Geometry: final body of the model. Coordinates: model frame, mm. A direction names the side the tool comes from. Coordinates: 2 decimals unless noted, no trailing zeros. Loops run counter-clockwise (first coordinate to the right, second up) from the corner with the lowest first, then second, coordinate; pieces in that order, holes last. Notation, with made-up numbers: (-40, 6) - (1, 6) arc R17 ccw to (1, 19) - close; hole circle Ø4 at (-10, -24). An arc over 180 degrees is marked (long way). Put each result on its own line as item: value. Start each with the question number.
1) Reachability of faces 4 (the flat face through (10, 3, 7)), 5 (the flat face through (20.5, 0, 8)), 6 (the flat face through (10, -3, 7)) from +Z, -Z, +X, -X, +Y, -Y: full face, straight path, thin tool, end or side. Return the list, or none.
2) Section B-B on x = 10. Output: boundary loops of the cut face in (y, z), and give its area (3 significant figures).
3) Section C-C on y = 0. Output: boundary loops of the cut face in (x, z), and give its area (3 significant figures).
4) Section A-A on z = 15. Output: boundary loops of the cut face in (x, y), and give its area (3 significant figures).
5) Section D-D on z = 9.5. Output: boundary loops of the cut face in (x, y), and give its area (3 significant figures).
6) Draft query along X for faces 1 (the cylindrical face through (13.502, -9.715, 0.301)), 2 (the cylindrical face through (28.58, 0.78, 2.54)), 3 (the flat face through (31.5, 0, 2)). Return one class per face: +X half, -X half, draft (parallel to the pull), parting line (faces both ways), or undercut.
7) Material intervals for line 1 along Y through (x, z) = (10, 3.5); line 2 along Z through (x, y) = (-2.95, 0); line 3 along X through (y, z) = (2, 12.25), sorted ascending. Write a range as from..to.
8) Contact query for flat-ended pins moving along their axis: pin 1 Ø4 at (y, z) = (2.5, 18.5) entering from +X; pin 2 Ø5 at (x, y) = (6, 0.5) entering from +Z; pin 3 Ø8 at (x, z) = (15, 11.5) entering from -Y; pin 4 Ø4 at (x, y) = (10, 0) entering from -Z. Output: stop coordinate, or through.
```python
from build123d import *

# Parameters (mm, degrees)
F0_W      = 31.5
F0_H      = 20
F1_DEPTH  = 5
F2_W      = 31.5
F2_H      = 6
F3_DEPTH  = 5
F4_R      = 2.5
F5_DEPTH  = 25
F6_W      = 11.2
F6_H      = 6
F7_DEPTH  = 5
F8_R      = 2.6
F9_DEPTH  = 5
F10_R     = 2.6
F11_DEPTH = 4
F12_R     = 1


# Not quite as in the source:
# - a fillet or chamfer that OpenCascade refuses, or shapes differently, is made with other operations: its cross-section is extruded or revolved along the edge and cut away or added
# - a feature names something its author has since deleted; it is built from what else it names


with BuildPart() as f1:
    # F0 (on Top) → F1 (new body)
    with BuildSketch(Plane.XY):
        with Locations((15.75, 0)):
            Rectangle(F0_W, F0_H)
    extrude(amount=F1_DEPTH)

    # F2 (on face) → F3 (join)
    with BuildSketch(Plane.XY.offset(5)):
        with Locations((15.75, 0)):
            Rectangle(F2_W, F2_H)
    extrude(amount=F3_DEPTH)

    # F4 (on face) → F5 (cut)
    with BuildSketch(Plane.XY.offset(10)):
        with Locations((10, 0)):
            Circle(F4_R)
    extrude(amount=-F5_DEPTH, mode=Mode.SUBTRACT)

    # F6 (on face) → F7 (cut, through all)
    with BuildSketch(Plane.XY.offset(10)):
        with Locations((26.1, 0)):
            Rectangle(F6_W, F6_H)
    extrude(amount=-F7_DEPTH, mode=Mode.SUBTRACT)

    # F8 (on face) → F9 (cut, through all)
    with BuildSketch(Plane.XY.offset(5)):
        with Locations((26.1, 0)):
            Circle(F8_R)
    extrude(amount=-F9_DEPTH, mode=Mode.SUBTRACT)

    # F10 (on face) → F11 (join)
    with BuildSketch(Plane(origin=(0, 0, 0), x_dir=(0, -1, 0), z_dir=(-1, 0, 0))):
        Polygon((-10, 25), (-10, 5), (-3, 5), (-3, 10), (3, 10), (3, 5), (10, 5), (10, 25), align=None)
        with Locations((0, 15)):
            Circle(F10_R, mode=Mode.SUBTRACT)
        Polygon((-10, 5), (-10, 0), (10, 0), (10, 5), (3, 5), (3, 10), (-3, 10), (-3, 5), align=None)
    extrude(amount=F11_DEPTH)

    # F12
    f12_edges = [f1.edges().sort_by_distance(p)[0] for p in [
        (-2, -10, 25),
        (-2, 10, 25),
        (13.75, -10, 0),
        (13.75, 10, 0),
    ]]
    fillet(f12_edges, radius=F12_R)

    # F13: chamfer of 0.5 x 0.2886751346 on 1 edges, made by hand

    # F13_s1 → F13_t2 (revolve, cut)
    with BuildSketch(Plane.XZ):
        Polygon((12.7886751346, 0), (12.5, 0.5), (12.5, 0), align=None)
    revolve(axis=Axis((10, 0, 0), (0, 0, 1)), mode=Mode.SUBTRACT)


solid = f1.part
```
Answer block:
1. face 4: +Z, +X, +Y
1. face 5: +Z, +X, +Y, -Y
1. face 6: +Z, +X, -Y
2. outline: (-10, 1) arc R1 ccw to (-9, 0) - (-2.79, 0) - (-2.5, 0.5) - (-2.5, 10) - (-3, 10) - (-3, 5) - (-10, 5) - close; (2.5, 0.5) - (2.79, 0) - (9, 0) arc R1 ccw to (10, 1) - (10, 5) - (3, 5) - (3, 10) - (2.5, 10) - close
2. area: 79.4 mm²
3. outline: (-4, 0) - (7.21, 0) - (7.5, 0.5) - (7.5, 10) - (0, 10) - (0, 12.4) - (-4, 12.4) - close; (-4, 17.6) - (0, 17.6) - (0, 25) - (-4, 25) - close; (12.5, 0.5) - (12.79, 0) - (23.5, 0) - (23.5, 5) - (20.5, 5) - (20.5, 10) - (12.5, 10) - close; (28.7, 0) - (31.5, 0) - (31.5, 5) - (28.7, 5) - close
3. area: 263 mm²
4. outline: (-4, -10) - (0, -10) - (0, -2.6) - (-4, -2.6) - close; (-4, 2.6) - (0, 2.6) - (0, 10) - (-4, 10) - close
4. area: 59.2 mm²
5. outline: (-4, -10) - (0, -10) - (0, -3) - (20.5, -3) - (20.5, 3) - (0, 3) - (0, 10) - (-4, 10) - close; hole circle Ø5 at (10, 0)
5. area: 183 mm²
6. face 1: draft
6. face 2: undercut
6. face 3: +X half
7. line 1: y = -10..-2.5, 2.5..10
7. line 2: z = 0..12.4, 17.6..25
7. line 3: x = -4..0
8. pin 1: stops at x = 0
8. pin 2: stops at z = 10
8. pin 3: stops at y = -3
8. pin 4: passes through
